The figure shows three views and two pictorial views of one solid part (mm, origin at its lowest corner). Answer the questions. A direction names the side the tool comes from. Round coordinates to 2 decimals unless told otherwise and drop trailing zeros. Order: outer loops, then holes, each group sorted by start corner. A loop starts at its lowest first (then second) coordinate and runs counter-clockwise, first axis right, second up. Notation, with made-up numbers: (30, 0.25) -> (85, 0.25) arc R13 cw to (85, 19.25) -> close; hole circle Ø6 at (59, 47). An arc over 180 degrees is marked (long way). One line per item, written item: value. Start each with the question number.
1. Section A-A (x = 9) is taken. Give the vertices of the cut face in (y, z).
2. For the marked faces 5 and 6, determine the directions among +Z, -Z, +X, -X, +Y, -Y from which every point of the face is accessible in a straight line to the end or side of a thin tool.
3. Section D-D (x = 25) is taken. Give the vertices of the cut face in (y, z).
4. Section C-C (y = 15) is taken. Give the vertices of the cut face in (x, z), then the cut area to 3 significant figures.
5. The mould has two halves that part along Z. Classify the marked faces 1, 2, 3 and 4: released by +Z, released by -Z, zero draft, split by the parting line, or undercut.
6. Consider line 1 (X direction, y = 5, z = 11); line 2 (Y direction, x = 25, z = 1.55); line 3 (Z direction, x = 12, y = 20.25). Determine where each line is inside the solid, lowest interval first.
7. Section B-B (z = 22.5) is taken. Give the vertices of the cut face in (x, y).
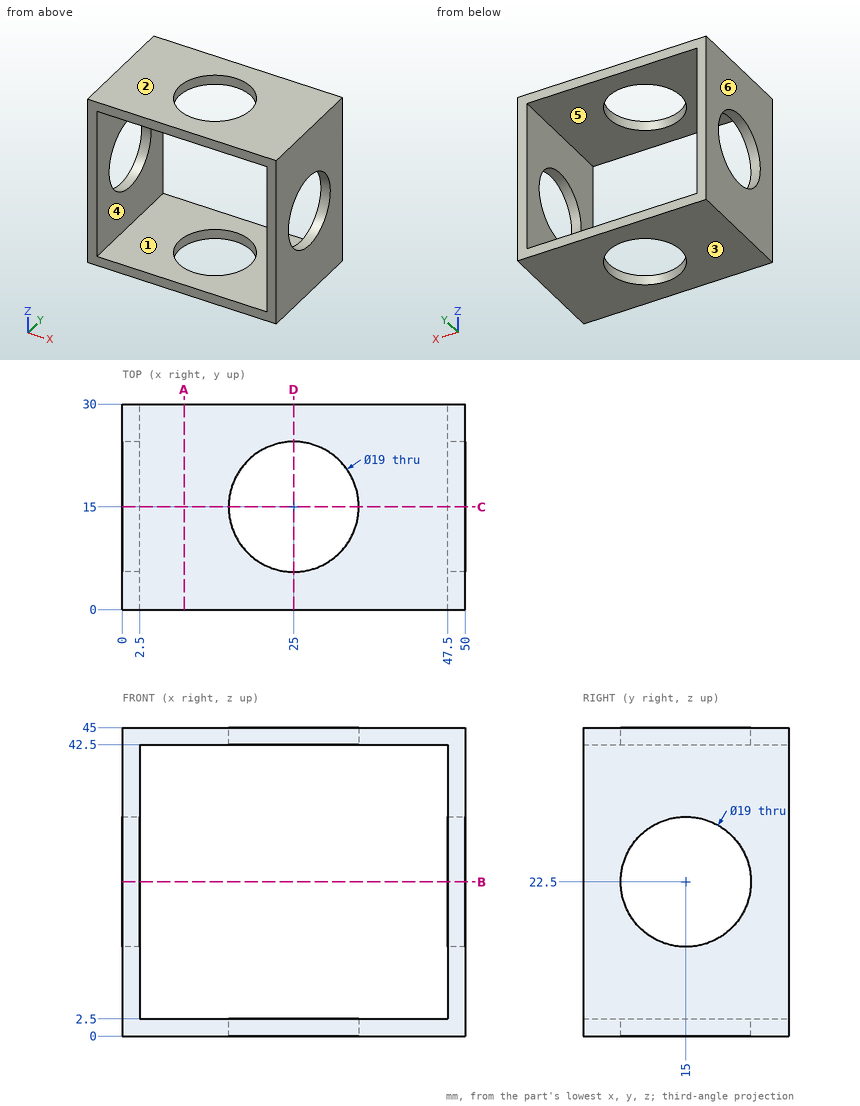
Answer:
1. outline: (0, 0) -> (30, 0) -> (30, 2.5) -> (0, 2.5) -> close; (0, 42.5) -> (30, 42.5) -> (30, 45) -> (0, 45) -> close
2. face 5: +Y, -Y
2. face 6: +Z, -Z, -X, +Y, -Y
3. outline: (0, 0) -> (5.5, 0) -> (5.5, 2.5) -> (0, 2.5) -> close; (0, 42.5) -> (5.5, 42.5) -> (5.5, 45) -> (0, 45) -> close; (24.5, 0) -> (30, 0) -> (30, 2.5) -> (24.5, 2.5) -> close; (24.5, 42.5) -> (30, 42.5) -> (30, 45) -> (24.5, 45) -> close
4. outline: (0, 0) -> (15.5, 0) -> (15.5, 2.5) -> (2.5, 2.5) -> (2.5, 13) -> (0, 13) -> close; (0, 32) -> (2.5, 32) -> (2.5, 42.5) -> (15.5, 42.5) -> (15.5, 45) -> (0, 45) -> close; (34.5, 0) -> (50, 0) -> (50, 13) -> (47.5, 13) -> (47.5, 2.5) -> (34.5, 2.5) -> close; (34.5, 42.5) -> (47.5, 42.5) -> (47.5, 32) -> (50, 32) -> (50, 45) -> (34.5, 45) -> close
4. area: 260 mm^2
5. face 1: undercut
5. face 2: released by +Z
5. face 3: released by -Z
5. face 4: undercut
6. line 1: 0 to 2.5, 47.5 to 50
6. line 2: 0 to 5.5, 24.5 to 30
6. line 3: 0 to 2.5, 42.5 to 45
7. outline: (0, 0) -> (2.5, 0) -> (2.5, 5.5) -> (0, 5.5) -> close; (0, 24.5) -> (2.5, 24.5) -> (2.5, 30) -> (0, 30) -> close; (47.5, 0) -> (50, 0) -> (50, 5.5) -> (47.5, 5.5) -> close; (47.5, 24.5) -> (50, 24.5) -> (50, 30) -> (47.5, 30) -> close
